Check sheet for the drawn part. Datum: minimum x, y, z corner. Units: mm. Give positions to 0.01 mm unless a question says otherwise; leave off trailing zeros. Loops run counter-clockwise (first coordinate to the right, second up) from the corner with the lowest first, then second, coordinate; pieces in that order, holes last. Notation, with made-up numbers: (58.5, 79) - (114.5, 79) arc R22 ccw to (114.5, 111) - close; hole circle Ø3 at (-22, -9). An arc over 180 degrees is marked (long way). Use one line per item in the form item = value.
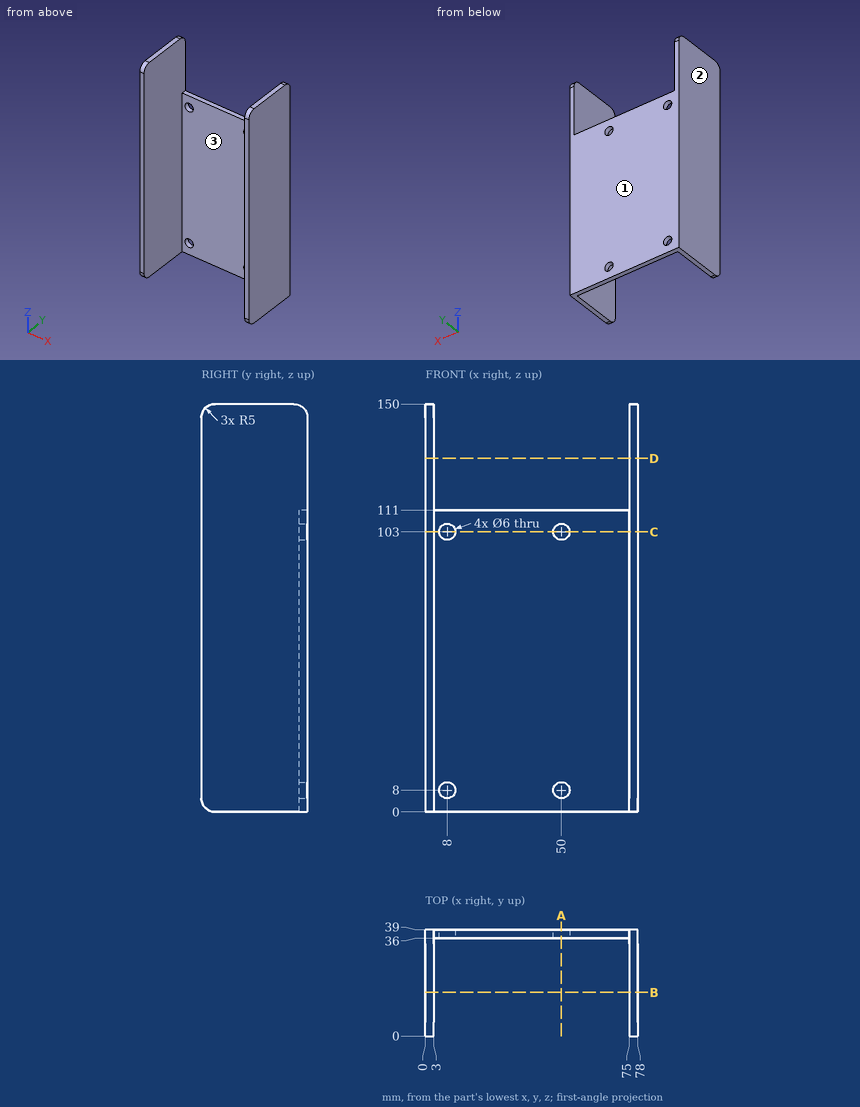
1. Depth check by flat-ended pin: pin 1 Ø1 at (y, z) = (9.5, 17.5) entering from -X; pin 2 Ø1.5 at (x, y) = (51, 38) entering from +Z; pin 3 Ø8 at (x, z) = (8, 8) entering from -Y. Enter the tip coordinate at first touch or a pass-through.
Result set:
pin_1 = 0
pin_2 = 111
pin_3 = 36
2. Scan lines: probe 1 along Z at (x, y) = (8, 38.15); probe 2 along X at (y, z) = (38, 8); probe 3 along X at (y, z) = (35, 25). Record each from-to range of solid material in increasing order.
Result set:
probe_1 = 0 to 5, 11 to 100, 106 to 111
probe_2 = 0 to 5, 11 to 47, 53 to 78
probe_3 = 0 to 3, 75 to 78
3. Section check C-C, the plane z = 103. Record the cut outline in (x, y).
Result set:
outline = (0, 0) - (3, 0) - (3, 36) - (5, 36) - (5, 39) - (0, 39) - close; (11, 36) - (47, 36) - (47, 39) - (11, 39) - close; (53, 36) - (75, 36) - (75, 0) - (78, 0) - (78, 39) - (53, 39) - close
4. Section check D-D, the plane z = 130. Record the cut outline in (x, y), then the cut area to 3 significant figures.
Result set:
outline = (0, 0) - (3, 0) - (3, 39) - (0, 39) - close; (75, 0) - (78, 0) - (78, 39) - (75, 39) - close
area = 234 mm²
5. Draft check along X on the marked faces 1, 2 and 3. Enter one of: released by +X, released by -X, zero draft, split by the parting line, or undercut.
Result set:
face_1 = zero draft
face_2 = released by -X
face_3 = undercut
6. Section check B-B, the plane y = 16. Record the cut outline in (x, z), then the cut area to 3 significant figures.
Result set:
outline = (0, 0) - (3, 0) - (3, 150) - (0, 150) - close; (75, 0) - (78, 0) - (78, 150) - (75, 150) - close
area = 900 mm²
7. Section check A-A, the plane x = 50. Record the cut outline in (y, z), then the cut area to 3 significant figures.
Result set:
outline = (36, 0) - (39, 0) - (39, 5) - (36, 5) - close; (36, 11) - (39, 11) - (39, 100) - (36, 100) - close; (36, 106) - (39, 106) - (39, 111) - (36, 111) - close
area = 297 mm²
